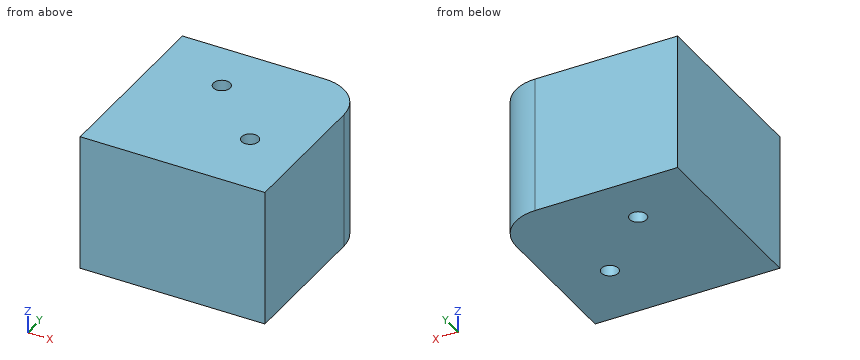
from build123d import *

# Parameters (mm, degrees)
SKETCH_W     = 35
SKETCH_H     = 35
PAD_DEPTH    = 26
SKETCH001_R  = 1.6
POCKET_DEPTH = 26.001
FILLET_R     = 8


with BuildPart() as part:
    # Sketch → Pad (new body)
    with BuildSketch(Plane.XY):
        with Locations((17.5, 17.5)):
            Rectangle(SKETCH_W, SKETCH_H)
    extrude(amount=PAD_DEPTH)

    # Sketch001 (on Face6 of Pad) → Pocket (cut, through all)
    with BuildSketch(Plane.XY.offset(26)):
        with Locations((25, 13)):
            Circle(SKETCH001_R)
        with Locations((13, 25)):
            Circle(SKETCH001_R)
    extrude(amount=-POCKET_DEPTH, mode=Mode.SUBTRACT)

    # Fillet
    fillet_edges = [part.edges().sort_by_distance(p)[0] for p in [
        (35, 35, 13),
    ]]
    fillet(fillet_edges, radius=FILLET_R)


solid = part.part
The model under review builds one solid part; all positions refer to its coordinate system, in mm. Round coordinates to 2 decimals unless told otherwise and drop trailing zeros. Loops run counter-clockwise (first coordinate to the right, second up) from the corner with the lowest first, then second, coordinate; pieces in that order, holes last. Notation, with made-up numbers: (-20, 12.25) -> (-10, 12.25) arc R34 ccw to (-10, 46.25) -> close; hole circle Ø10 at (-32, 68). An arc over 180 degrees is marked (long way). Write item = value, one per line. Start each with the question number.
Item 1: To check wall thickness, follow L1, parallel to Y at x = 25, z = 11; L2, parallel to Y at x = 13, z = 6.5; L3, parallel to X at y = 24, z = 22.5. State the ranges of each line that lie inside material, in increasing order.
Item 2: Take a section at A-A on y = 25. Give the boundary of the cut face in (x, z), plus the area to 3 significant figures.
Item 3: Take a section at D-D on x = 30.5. Give the boundary of the cut face in (y, z), plus the area to 3 significant figures.
Item 4: Take a section at B-B on z = 13.25. Give the boundary of the cut face in (x, y), plus the area to 3 significant figures.
Result:
q1.L1 = 0 to 11.4, 14.6 to 35
q1.L2 = 0 to 23.4, 26.6 to 35
q1.L3 = 0 to 11.75, 14.25 to 35
q2.outline = (0, 0) -> (11.4, 0) -> (11.4, 26) -> (0, 26) -> close; (14.6, 0) -> (35, 0) -> (35, 26) -> (14.6, 26) -> close
q2.area = 827 mm²
q3.outline = (0, 0) -> (34.19, 0) -> (34.19, 26) -> (0, 26) -> close
q3.area = 889 mm²
q4.outline = (0, 0) -> (35, 0) -> (35, 27) arc R8 ccw to (27, 35) -> (0, 35) -> close; hole circle Ø3.2 at (13, 25); hole circle Ø3.2 at (25, 13)
q4.area = 1,200 mm²
